Can you work these out from the model? Positions are in its coordinate system, mm. A direction names the side the tool comes from. Give positions to 0.01 mm unless a question says otherwise; leave off trailing zeros. Write each loop counter-clockwise with the first axis right and the second up, starting at its lowest first coordinate (ties: lowest second). Pieces come first, ordered by that corner, then holes. Notation, with made-up numbers: (-17, 9) - (17, 9) arc R25 cw to (17, 40) - close; hole circle Ø6 at (-14, -11). An arc over 180 degrees is marked (long way). Return JSON: item names as keys, results as strings. Group by question number.
from build123d import *

# Parameters (mm, degrees)
BOSS_EXTRUDE1_DEPTH = 40
CUT_EXTRUDE1_DEPTH  = 40
SKETCH3_W           = 20
SKETCH3_H           = 20
CUT_EXTRUDE2_DEPTH  = 20
BOSS_EXTRUDE4_DEPTH = 20
CUT_EXTRUDE3_DEPTH  = 20


with BuildPart() as part:
    # Sketch1 → Boss-Extrude1 (new body)
    with BuildSketch(Plane.XY):
        Polygon((0, 0), (0, 40), (20, 40), (20, 20), (40, 20), (40, 0), align=None)
    extrude(amount=BOSS_EXTRUDE1_DEPTH)

    # Sketch2 → Cut-Extrude1 (cut)
    with BuildSketch(Plane(origin=(0, 0, 0), x_dir=(-1, 0, 0), z_dir=(0, -1, 0))):
        with BuildLine():
            Line((0, -40), (0, -20))
            ThreePointArc((0, -20), (-5.857864376, -34.142135624), (-20, -40))
            Line((-20, -40), (0, -40))
        make_face()
        with BuildLine():
            Line((-40, -40), (-20, -40))
            ThreePointArc((-20, -40), (-34.142135624, -34.142135624), (-40, -20))
            Line((-40, -20), (-40, -40))
        make_face()
    extrude(amount=-CUT_EXTRUDE1_DEPTH, mode=Mode.SUBTRACT)

    # Sketch3 → Cut-Extrude2 (cut)
    with BuildSketch(Plane(origin=(0, 20, 0), x_dir=(1, 0, 0), z_dir=(0, 1, 0))):
        with Locations((10, -10)):
            Rectangle(SKETCH3_W, SKETCH3_H)
    extrude(amount=CUT_EXTRUDE2_DEPTH, mode=Mode.SUBTRACT)

    # Sketch4 → Boss-Extrude4 (add)
    with BuildSketch(Plane(origin=(0, 20, 0), x_dir=(1, 0, 0), z_dir=(0, 1, 0))):
        with BuildLine():
            Line((20, 0), (40, 0))
            Line((40, 0), (40, -20))
            ThreePointArc((40, -20), (25.857864376, -14.142135624), (20, 0))
        make_face()
    extrude(amount=BOSS_EXTRUDE4_DEPTH)

    # Sketch5 → Cut-Extrude3 (cut)
    with BuildSketch(Plane(origin=(0, 40, 0), x_dir=(1, 0, 0), z_dir=(0, 1, 0))):
        with BuildLine():
            ThreePointArc((0, -20), (5.857864376, -34.142135624), (20, -40))
            Line((20, -40), (20, -20))
            Line((20, -20), (0, -20))
        make_face()
    extrude(amount=-CUT_EXTRUDE3_DEPTH, mode=Mode.SUBTRACT)

    # Sketch6 → Cut-Revolve1 (revolve, cut)
    with BuildSketch(Plane.ZY):
        Polygon((0, 0), (20, 20), (0, 20), align=None)
    revolve(axis=Axis((0, 0, 0), (0, 1, 0)), mode=Mode.SUBTRACT)


solid = part.part
1) Imagine slicing it at C-C, the plane z = 21. Write out the boundary of the cut face in (x, y), and give its area (3 significant figures).
2) Imagine slicing it at A-A, the plane y = 11. Write out the boundary of the cut face in (x, z), and give its area (3 significant figures).
3) On a 3-axis mill with a long thin cutter (end or side, diameter ignored), from which of +Z, -Z, +X, -X, +Y, -Y can I reach the whole of each face in a straight line? I mean faces 1 (the face through (0, 5, 14)), 2 (the face through (20, 20, 24)). Say none if no direction works.
4) Imagine slicing it at D-D, the plane y = 21. Write out the boundary of the cut face in (x, z).
5) Imagine slicing it at B-B, the plane x = 36.5. Write out the boundary of the cut face in (y, z).
6) I need wall thicknesses on line 1 along Y through (x, z) = (14.5, 36.5); line 2 along Z through (x, y) = (18, 4); line 3 along Z through (x, y) = (29, 14). Which ranges of each line are inside material? Lowest first, please.
7) Will these pins go through, and if not, where does the flat tip stop? pin 1 Ø1 at (x, z) = (20.5, 30.5) entering from +Y; pin 2 Ø1 at (y, z) = (18, 31.5) entering from -X.
Resolved:
{
 "1": {"outline": "(0.03, 0) - (39.97, 0) - (39.97, 20) - (0.03, 20) - close", "area": "799 mm^2"},
 "2": {"outline": "(0, 11) arc R11 cw to (11, 0) - (40, 0) - (40, 20) arc R20 ccw to (0, 20) - close", "area": "1,330 mm^2"},
 "3": {"face 1": "+Z, -Z, -X, +Y, -Y", "face 2": "+Z, -X, +Y"},
 "4": {"outline": "(20, 0) - (40, 0) - (40, 20) arc R20 ccw to start"},
 "5": {"outline": "(0, 0) - (40, 0) - (40, 19.69) - (20, 19.69) - (20, 31.3) - (0, 31.3) - close"},
 "6": {"line 1": "0 to 20", "line 2": "0 to 39.9", "line 3": "0 to 37.86"},
 "7": {"pin 1": "y = 20", "pin 2": "x = 3.3"}
}
